Verification items for this drawing (mm, ordinates from the low corner). Coordinates: 2 decimals unless noted, no trailing zeros. Write each loop counter-clockwise with the first axis right and the second up, starting at its lowest first coordinate (ties: lowest second). Pieces come first, ordered by that corner, then holes.
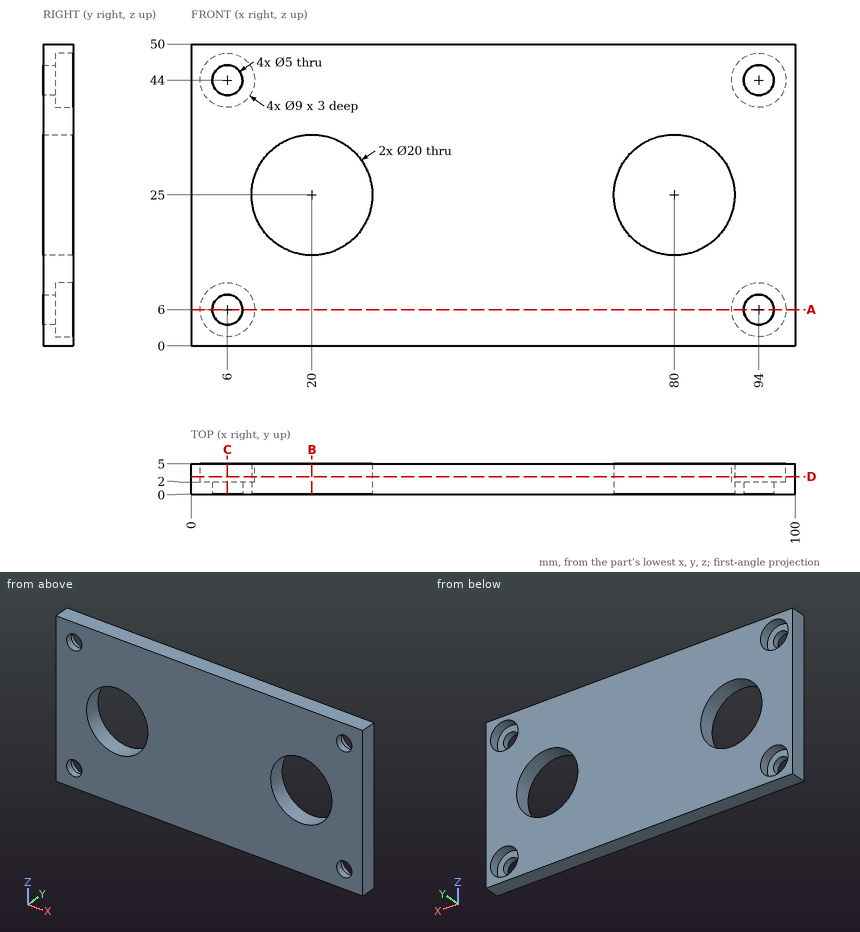
1. Sectioned sample at C-C, the plane x = 6. Record the boundary of the cut face in (y, z), and give its area (3 significant figures).
Computed values:
outline: (0, 0) - (5, 0) - (5, 1.5) - (2, 1.5) - (2, 3.5) - (0, 3.5) - close; (0, 8.5) - (2, 8.5) - (2, 10.5) - (5, 10.5) - (5, 39.5) - (2, 39.5) - (2, 41.5) - (0, 41.5) - close; (0, 46.5) - (2, 46.5) - (2, 48.5) - (5, 48.5) - (5, 50) - (0, 50) - close
area: 176 mm2
2. Thickness scan on line 1 along X through (y, z) = (3.9, 44); line 2 along X through (y, z) = (0.6, 44); line 3 along Z through (x, y) = (6, 1.1). Record the ranges inside material, lowest first.
Computed values:
line 1: x = 0 to 1.5, 10.5 to 89.5, 98.5 to 100
line 2: x = 0 to 3.5, 8.5 to 91.5, 96.5 to 100
line 3: z = 0 to 3.5, 8.5 to 41.5, 46.5 to 50
3. Sectioned sample at B-B, the plane x = 20. Record the boundary of the cut face in (y, z), and give its area (3 significant figures).
Computed values:
outline: (0, 0) - (5, 0) - (5, 15) - (0, 15) - close; (0, 35) - (5, 35) - (5, 50) - (0, 50) - close
area: 150 mm2
4. Sectioned sample at A-A, the plane z = 6. Record the boundary of the cut face in (x, y).
Computed values:
outline: (0, 0) - (3.5, 0) - (3.5, 2) - (1.5, 2) - (1.5, 5) - (0, 5) - close; (8.5, 0) - (91.5, 0) - (91.5, 2) - (89.5, 2) - (89.5, 5) - (10.5, 5) - (10.5, 2) - (8.5, 2) - close; (96.5, 0) - (100, 0) - (100, 5) - (98.5, 5) - (98.5, 2) - (96.5, 2) - close
5. Sectioned sample at D-D, the plane y = 2.9. Record the boundary of the cut face in (x, z).
Computed values:
outline: (0, 0) - (100, 0) - (100, 50) - (0, 50) - close; hole circle Ø9 at (6, 6); hole circle Ø9 at (6, 44); hole circle Ø20 at (20, 25); hole circle Ø20 at (80, 25); hole circle Ø9 at (94, 6); hole circle Ø9 at (94, 44)
6. Gauge pin test, flat ends, axial feed: pin 1 Ø14.5 at (x, z) = (94, 6) entering from +Y; pin 2 Ø7 at (x, z) = (94, 44) entering from +Y; pin 3 Ø4 at (x, z) = (6, 6) entering from -Y. Record the tip position at first contact, or that the pin passes through.
Computed values:
pin 1: stops at y = 5
pin 2: stops at y = 2
pin 3: passes through
